```python
from build123d import *

# Parameters (mm, degrees)
SKETCH1_W           = 20.5
SKETCH1_H           = 20.5
SKETCH1_R           = 1.25
BOSS_EXTRUDE1_DEPTH = 2
SKETCH2_W           = 20.5
SKETCH2_H           = 2.5
BOSS_EXTRUDE2_DEPTH = 12


with BuildPart() as part:
    # Sketch1 → Boss-Extrude1 (new body)
    with BuildSketch(Plane(origin=(0, 0, 0), x_dir=(0, 0, -1), z_dir=(1, 0, 0))):
        Rectangle(SKETCH1_W, SKETCH1_H)
        with Locations((-7.5, 7.5)):
            Circle(SKETCH1_R, mode=Mode.SUBTRACT)
        with Locations((7.5, 7.5)):
            Circle(SKETCH1_R, mode=Mode.SUBTRACT)
    extrude(amount=BOSS_EXTRUDE1_DEPTH)

    # Sketch2 → Boss-Extrude2 (add)
    with BuildSketch(Plane.ZY):
        with Locations((0, -9)):
            Rectangle(SKETCH2_W, SKETCH2_H)
    extrude(amount=BOSS_EXTRUDE2_DEPTH)


solid = part.part
```
Source: CAD feature listing. Evaluate the final solid. Frame: model axes, mm. A direction names the side the tool comes from. Give positions to 0.01 mm unless a question says otherwise; leave off trailing zeros. Order: outer loops, then holes, each group sorted by start corner. A loop starts at its lowest first (then second) coordinate and runs counter-clockwise, first axis right, second up. Notation, with made-up numbers: (-34.5, 10) -> (18.5, 10) arc R10 ccw to (18.5, 14) -> close; hole circle Ø5 at (-38, 28). An arc over 180 degrees is marked (long way). Use a Markdown table: item, result.
Q1. First-contact query: P1, Ø2, axis at y = 0, z = -3, coming from the -X side; P2, Ø3.5, axis at x = -3.5, z = 3.5, coming from the +Y side; P3, Ø1.5, axis at y = 7.5, z = 7.5, coming from the -X side. Flat tips, straight axial feed; report the tip coordinate or a pass-through.
A:
| item | result |
|---|---|
| P1 | x = 0 |
| P2 | y = -7.75 |
| P3 | through |
Q2. Access query for faces 5 (the face through (-6, -7.75, 0)), 6 (the face through (-5, -10.25, 0)). Directions: +Z, -Z, +X, -X, +Y, -Y. A direction counts if a zero-diameter tool reaches every point of the face in a straight line with its end or side. Return the directions, or none.
A:
| item | result |
|---|---|
| face 5 | +Z, -Z, -X, +Y |
| face 6 | +Z, -Z, +X, -X, -Y |
Q3. Section B-B (z = -7.5). Return the cut outline in (x, y).
A:
| item | result |
|---|---|
| outline | (-12, -10.25) -> (2, -10.25) -> (2, 6.25) -> (0, 6.25) -> (0, -7.75) -> (-12, -7.75) -> close; (0, 8.75) -> (2, 8.75) -> (2, 10.25) -> (0, 10.25) -> close |
Q4. Pull-direction query (Z, two-part tool) for faces 1 (the face through (1, -4, -10.25)), 2 (the face through (0.99, 7.55, -6.25)), 3 (the face through (-12, -9, 0)), 4 (the face through (1, -4, 10.25)); classes: +Z half, -Z half, draft (parallel to the pull), parting line (faces both ways), or undercut.
A:
| item | result |
|---|---|
| face 1 | -Z half |
| face 2 | undercut |
| face 3 | draft |
| face 4 | +Z half |
Q5. Material intervals for line 1 (Y direction, x = 0.9, z = 7.5); line 2 (X direction, y = -6, z = -1.5); line 3 (Y direction, x = -1.5, z = -4.75), sorted ascending. Write a range as [from, to].
A:
| item | result |
|---|---|
| line 1 | [-10.25, 6.25], [8.75, 10.25] |
| line 2 | [0, 2] |
| line 3 | [-10.25, -7.75] |
Q6. Section D-D (x = -8). Return the cut outline in (y, z).
A:
| item | result |
|---|---|
| outline | (-10.25, -10.25) -> (-7.75, -10.25) -> (-7.75, 10.25) -> (-10.25, 10.25) -> close |
Q7. Section A-A (y = 7.5). Return the cut outline in (x, z).
A:
| item | result |
|---|---|
| outline | (0, -10.25) -> (2, -10.25) -> (2, -8.75) -> (0, -8.75) -> close; (0, -6.25) -> (2, -6.25) -> (2, 6.25) -> (0, 6.25) -> close; (0, 8.75) -> (2, 8.75) -> (2, 10.25) -> (0, 10.25) -> close |
Q8. Section C-C (z = 9.25). Return the cut outline in (x, y), and give its area (3 significant figures).
A:
| item | result |
|---|---|
| outline | (-12, -10.25) -> (2, -10.25) -> (2, 10.25) -> (0, 10.25) -> (0, -7.75) -> (-12, -7.75) -> close |
| area | 71.0 mm^2 |
